```python
from build123d import *

# Parameters (mm, degrees)
SKETCH1_R           = 20
BOSS_EXTRUDE1_DEPTH = 284
SKETCH2_W           = 99.610894942
SKETCH2_H           = 80
BOSS_EXTRUDE2_DEPTH = 10
FILLET1_R           = 2
FILLET2_R           = 1


with BuildPart() as part:
    # Sketch1 → Boss-Extrude1 (new body)
    with BuildSketch(Plane.XY):
        Circle(SKETCH1_R)
    extrude(amount=BOSS_EXTRUDE1_DEPTH)

    # Sketch2 → Boss-Extrude2 (add)
    with BuildSketch(Plane.XY.offset(284)):
        Rectangle(SKETCH2_W, SKETCH2_H)
    extrude(amount=BOSS_EXTRUDE2_DEPTH)

    # Fillet1
    fillet1_edges = [part.edges().sort_by_distance(p)[0] for p in [
        (-20, 0, 0),
    ]]
    fillet(fillet1_edges, radius=FILLET1_R)

    # Fillet2
    fillet2_edges = [part.edges().sort_by_distance(p)[0] for p in [
        (49.805447471, 0, 284),
        (49.805447471, -40, 289),
        (0, 40, 284),
        (49.805447471, 40, 289),
        (-49.805447471, 0, 284),
        (-49.805447471, 40, 289),
        (0, -40, 284),
        (-49.805447471, -40, 289),
        (49.805447471, 0, 294),
        (0, 40, 294),
        (-49.805447471, 0, 294),
        (0, -40, 294),
    ]]
    fillet(fillet2_edges, radius=FILLET2_R)


solid = part.part
```
Here's how the part is built. I have some questions about the finished solid (model axes, mm). A direction names the side the tool comes from. Give positions to 0.01 mm unless a question says otherwise; leave off trailing zeros. Write each loop counter-clockwise with the first axis right and the second up, starting at its lowest first coordinate (ties: lowest second). Pieces come first, ordered by that corner, then holes. Notation, with made-up numbers: (68, 79.25) -> (102, 79.25) arc R27 ccw to (102, 105.25) -> close; hole circle Ø3 at (-24, -7). An arc over 180 degrees is marked (long way). Write each question's results on one line, items separated by ' | '.
Item 1: If I drill on L1, parallel to Z at x = 43.5, y = 3.5; L2, parallel to X at y = -1.5, z = 97; L3, parallel to Y at x = 9.5, z = 191.5, over which ranges is the centre line in solid material (lowest first)?
Output:
L1: z = 284 to 294 | L2: x = -19.94 to 19.94 | L3: y = -17.6 to 17.6
Item 2: Suppose I cut it at C-C on z = 23.5. Write out the boundary of the cut face in (x, y).
Output:
outline: circle Ø40 at (0, 0)
Item 3: Suppose I cut it at A-A on y = 23. Write out the boundary of the cut face in (x, z).
Output:
outline: (-49.81, 285) arc R1 ccw to (-48.81, 284) -> (48.81, 284) arc R1 ccw to (49.81, 285) -> (49.81, 293) arc R1 ccw to (48.81, 294) -> (-48.81, 294) arc R1 ccw to (-49.81, 293) -> close
Item 4: For pin 1 Ø4 at (y, z) = (1, 261) entering from +X; pin 2 Ø4 at (y, z) = (-5.5, 153) entering from +X; pin 3 Ø8 at (y, z) = (10.5, 246.5) entering from +X, each with a flat end and sliding along its axis, tell me the tip position at first contact or that it passes through.
Output:
pin 1: stops at x = 20 | pin 2: stops at x = 19.69 | pin 3: stops at x = 18.91
Item 5: Suppose I cut it at B-B on x = 37. Write out the boundary of the cut face in (y, z), plus the area to 3 significant figures.
Output:
outline: (-40, 285) arc R1 ccw to (-39, 284) -> (39, 284) arc R1 ccw to (40, 285) -> (40, 293) arc R1 ccw to (39, 294) -> (-39, 294) arc R1 ccw to (-40, 293) -> close | area: 799 mm^2
Item 6: On a 3-axis mill with a long thin cutter (end or side, diameter ignored), from which of +Z, -Z, +X, -X, +Y, -Y can I reach the whole of each face in a straight line? I mean faces 1 (the face through (-49.805, -1, 289)), 2 (the face through (-4.336, -19.524, 141.026)). Say none if no direction works.
Output:
face 1: +Z, -Z, -X, +Y, -Y | face 2: -Z
Item 7: Suppose I cut it at D-D on y = 0. Write out the boundary of the cut face in (x, z), plus the area to 3 significant figures.
Output:
outline: (-49.81, 285) arc R1 ccw to (-48.81, 284) -> (-20, 284) -> (-20, 2) arc R2 ccw to (-18, 0) -> (18, 0) arc R2 ccw to (20, 2) -> (20, 284) -> (48.81, 284) arc R1 ccw to (49.81, 285) -> (49.81, 293) arc R1 ccw to (48.81, 294) -> (-48.81, 294) arc R1 ccw to (-49.81, 293) -> close | area: 12,400 mm^2
